Design review of the part shown in the three views and the two pictorial views. Dimensions are in mm from the part's minimum x, y and z. A direction names the side the tool comes from. Coordinates: 2 decimals unless noted, no trailing zeros. Order: outer loops, then holes, each group sorted by start corner. A loop starts at its lowest first (then second) coordinate and runs counter-clockwise, first axis right, second up. Notation, with made-up numbers: (15.5, -38.5) - (40.5, -38.5) arc R25 ccw to (40.5, -21.5) - close; hole circle Ø1 at (-26, 20.5). An arc over 180 degrees is marked (long way). One line per item, written item: value. Start each with the question number.
(1) For the marked faces 4 and 5, list the 3-axis set-ups (+Z, -Z, +X, -X, +Y, -Y) from which the entire face can be reached by the end or side of a thin tool; tool diameter is ignored.
(2) Consider section D-D on z = 12.5. Write out the cut boundary in (x, y).
(3) Consider section B-B on y = 7.5. Write out the cut boundary in (x, z).
(4) Consider section C-C on x = 11. Write out the cut boundary in (y, z), then the cut area to 3 significant figures.
(5) Mouldability with a two-part tool opening along X and no side actions: class the marked faces 1, 2 and 3 as released by +X, released by -X, zero draft, split by the parting line, or undercut.
(6) To check wall thickness, follow line 1 along X through (y, z) = (17, 22.5); line 2 along X through (y, z) = (12.25, 19.5); line 3 along Y through (x, z) = (63.5, 28.5). State the ranges of each line that lie inside material, in increasing order.
(7) Consider section A-A on z = 22.5. Write out the cut boundary in (x, y), then the cut area to 4 significant figures.
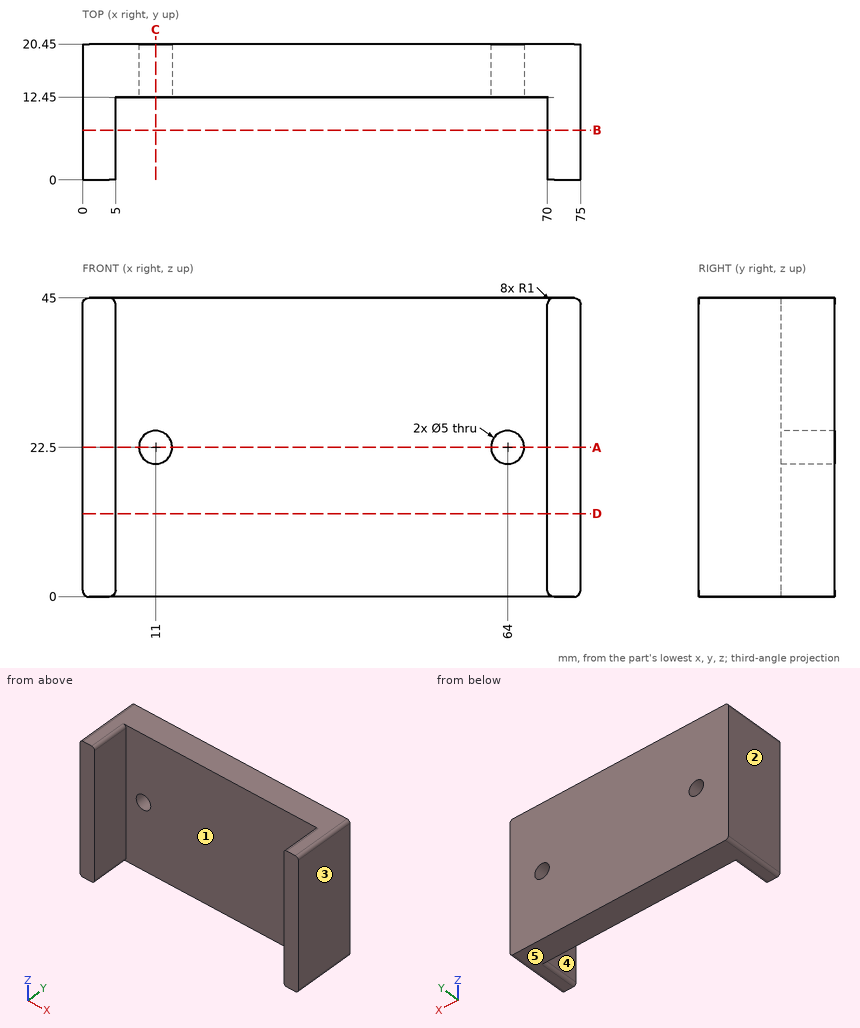
Geometry check:
1. face 4: +Z, -Z, -Y
1. face 5: -Z, +X, -X, +Y, -Y
2. outline: (0, 0) - (5, 0) - (5, 12.45) - (70, 12.45) - (70, 0) - (75, 0) - (75, 20.45) - (0, 20.45) - close
3. outline: (0, 1) arc R1 ccw to (1, 0) - (4, 0) arc R1 ccw to (5, 1) - (5, 44) arc R1 ccw to (4, 45) - (1, 45) arc R1 ccw to (0, 44) - close; (70, 1) arc R1 ccw to (71, 0) - (74, 0) arc R1 ccw to (75, 1) - (75, 44) arc R1 ccw to (74, 45) - (71, 45) arc R1 ccw to (70, 44) - close
4. outline: (12.45, 0) - (20.45, 0) - (20.45, 20) - (12.45, 20) - close; (12.45, 25) - (20.45, 25) - (20.45, 45) - (12.45, 45) - close
4. area: 320 mm^2
5. face 1: undercut
5. face 2: released by -X
5. face 3: released by +X
6. line 1: x = 0 to 8.5, 13.5 to 61.5, 66.5 to 75
6. line 2: x = 0 to 5, 70 to 75
6. line 3: y = 12.45 to 20.45
7. outline: (0, 0) - (5, 0) - (5, 12.45) - (8.5, 12.45) - (8.5, 20.45) - (0, 20.45) - close; (13.5, 12.45) - (61.5, 12.45) - (61.5, 20.45) - (13.5, 20.45) - close; (66.5, 12.45) - (70, 12.45) - (70, 0) - (75, 0) - (75, 20.45) - (66.5, 20.45) - close
7. area: 644.5 mm^2
